```python
from build123d import *

# Parameters (mm, degrees)
SKETCH1_R                 = 2
BOSS_EXTRUDE1_DEPTH       = 5
M2X0_4_TAPPED_HOLE1_D     = 1.6
M2X0_4_TAPPED_HOLE1_DEPTH = 2.999994
M2X0_4_TAPPED_HOLE1_TIP   = 0.480688495


with BuildPart() as part:
    # Sketch1 → Boss-Extrude1 (new body)
    with BuildSketch(Plane.XY):
        with BuildLine():
            Line((7.49299434, 88.359418723), (2.124641235, 98.779265156))
            Line((2.124641235, 98.779265156), (-10.502416807, 100.902673639))
            ThreePointArc((-10.502416807, 100.902673639), (-10.798602236, 98.463827502), (-10.342383239, 96.049793427))
            Line((-10.342383239, 96.049793427), (-9.053191571, 98.758664935))
            Line((-9.053191571, 98.758664935), (4.456621188, 88.438669077))
            ThreePointArc((4.456621188, 88.438669077), (3.787347561, 86.94932011), (3.73945192, 85.317206897))
            Line((3.73945192, 85.317206897), (6.070083914, 87.206162828))
            Line((6.070083914, 87.206162828), (7.49299434, 88.359418723))
        make_face()
        with Locations((0, 95.99791663)):
            Circle(SKETCH1_R, mode=Mode.SUBTRACT)
    extrude(amount=BOSS_EXTRUDE1_DEPTH)

    # M2x0.4 Tapped Hole1
    with Locations(Plane(origin=(16.212659079, 96.410176767, 0), x_dir=(0.986153532, -0.16583489, 0), z_dir=(0.16583489, 0.986153532, 0))):
        with Locations((-15.919803906, -2.5)):
            Hole(M2X0_4_TAPPED_HOLE1_D / 2, depth=M2X0_4_TAPPED_HOLE1_DEPTH)
            with Locations((0, 0, -(M2X0_4_TAPPED_HOLE1_DEPTH + M2X0_4_TAPPED_HOLE1_TIP / 2))):  # 118° drill point
                Cone(0, M2X0_4_TAPPED_HOLE1_D / 2, M2X0_4_TAPPED_HOLE1_TIP, mode=Mode.SUBTRACT)


solid = part.part
```
Geometry: final body of the model. Coordinates: model frame, mm. A direction names the side the tool comes from. Round coordinates to 2 decimals unless told otherwise and drop trailing zeros. Order: outer loops, then holes, each group sorted by start corner. A loop starts at its lowest first (then second) coordinate and runs counter-clockwise, first axis right, second up. Notation, with made-up numbers: (-25.5, -6) -> (-13.5, -6) arc R22 ccw to (-13.5, 32) -> close; hole circle Ø1 at (68, -24.5). An arc over 180 degrees is marked (long way). Write each question's results on one line, items separated by ' | '.
Q1. Access query for faces 4 (the face through (-9.7, 97.4, 2.5)), 5 (the face through (-10.8, 98.5, 2.5)). Directions: +Z, -Z, +X, -X, +Y, -Y. A direction counts if a zero-diameter tool reaches every point of the face in a straight line with its end or side. Return the directions, or none.
Response values:
face 4: +Z, -Z, -Y | face 5: +Z, -Z, -X
Q2. Ray query, line 1 along X through (y, z) = (97.75, 3.7); line 2 along X through (y, z) = (98, 2.1); line 3 along X through (y, z) = (96, 2.05). Return the intervals inside material, ascending.
Response values:
line 1: -10.74 to -9.53, -7.73 to -0.96, 0.96 to 2.65 | line 2: -10.77 to -9.41, -8.06 to -0.37, 1.04 to 2.53 | line 3: -5.44 to -2, 2 to 3.56
Q3. Section query C-C (x = 0). Count the separate pieces of the cut face and the enclosed holes in it, and give its area (3 significant figures).
Response values:
separate pieces: 3 | enclosed holes: 0 | area: 14.9 mm²
Q4. Pull-direction query (Y, two-part tool) for faces 1 (the face through (-2, 95, 5)), 2 (the face through (3.8, 87, 2.5)), 3 (the face through (-4.1, 99.826, 2.465)); classes: released by +Y, released by -Y, zero draft, split by the parting line, or undercut.
Response values:
face 1: zero draft | face 2: undercut | face 3: released by +Y
Q5. Section query B-B (y = 95.25). Output: boundary loops of the cut face in (x, z).
Response values:
outline: (-4.46, 0) -> (-1.85, 0) -> (-1.85, 5) -> (-4.46, 5) -> close; (1.85, 0) -> (3.94, 0) -> (3.94, 5) -> (1.85, 5) -> close
Q6. Section query A-A (z = 0.8). Output: boundary loops of the cut face in (x, y).
Response values:
outline: (-10.5, 100.9) arc R8.02 ccw to (-10.34, 96.05) -> (-9.05, 98.76) -> (4.46, 88.44) arc R4.18 ccw to (3.74, 85.32) -> (7.49, 88.36) -> (2.12, 98.78) -> close; hole circle Ø4 at (0, 96)
Q7. Section query D-D (z = 2.05). Output: boundary loops of the cut face in (x, y).
Response values:
outline: (-10.5, 100.9) arc R8.02 ccw to (-10.34, 96.05) -> (-9.05, 98.76) -> (4.46, 88.44) arc R4.18 ccw to (3.74, 85.32) -> (7.49, 88.36) -> (2.12, 98.78) -> (1.17, 98.94) -> (0.97, 97.75) arc R2 cw (long way) to (-0.34, 97.97) -> (-0.14, 99.16) -> close
